Geometry check sheet. Reference: drawing and pictorial views, mm from the part's lowest x, y, z. A direction names the side the tool comes from. Coordinates: 2 decimals unless noted, no trailing zeros. Write each loop counter-clockwise with the first axis right and the second up, starting at its lowest first coordinate (ties: lowest second). Pieces come first, ordered by that corner, then holes. Notation, with made-up numbers: (75, 39.5) -> (127, 39.5) arc R8 cw to (127, 46.5) -> close; hole circle Ø1 at (64.25, -30). An arc over 180 degrees is marked (long way). Use a Markdown table: item, result.
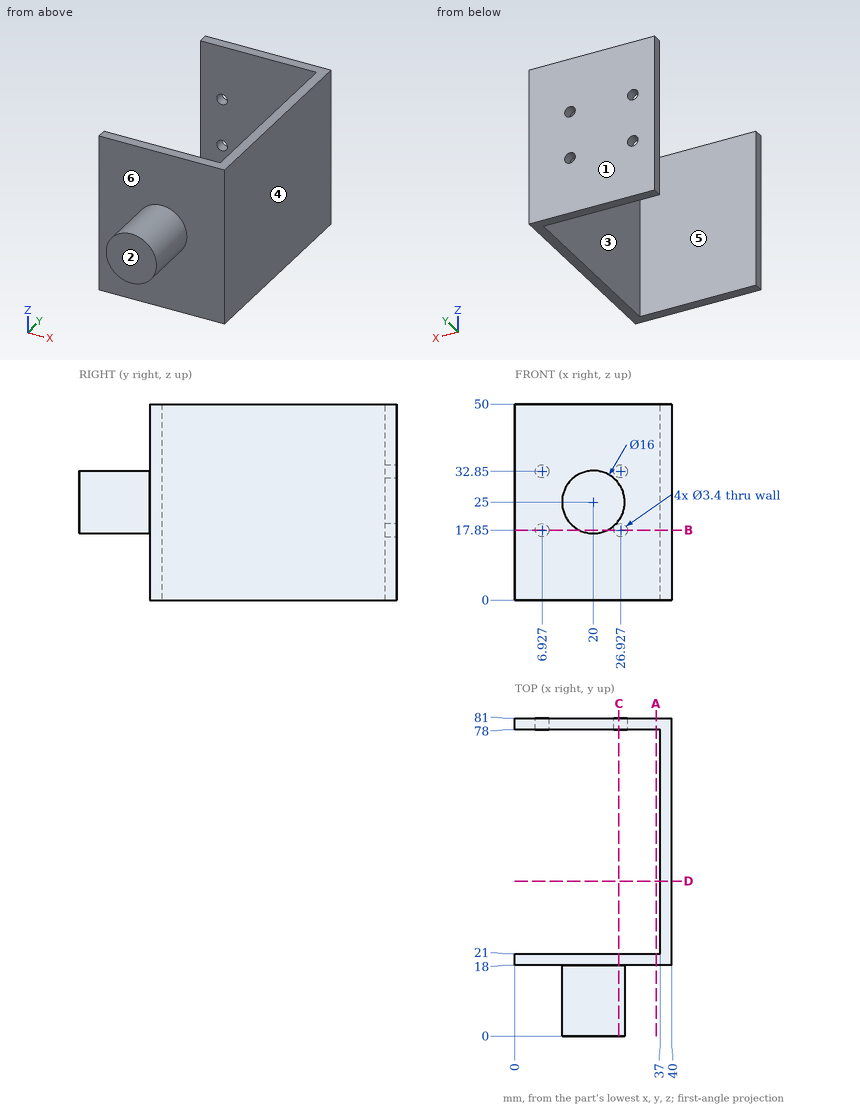
Item 1: Section check A-A on x = 36. Record the boundary of the cut face in (y, z), then the cut area to 3 significant figures.
Answer block:
| item | result |
|---|---|
| outline | (18, 0) -> (21, 0) -> (21, 50) -> (18, 50) -> close; (78, 0) -> (81, 0) -> (81, 50) -> (78, 50) -> close |
| area | 300 mm^2 |
Item 2: Section check C-C on x = 26.5. Record the boundary of the cut face in (y, z) (1 decimal).
Answer block:
| item | result |
|---|---|
| outline | (0, 20.3) -> (18, 20.3) -> (18, 0) -> (21, 0) -> (21, 50) -> (18, 50) -> (18, 29.7) -> (0, 29.7) -> close; (78, 0) -> (81, 0) -> (81, 16.2) -> (78, 16.2) -> close; (78, 19.5) -> (81, 19.5) -> (81, 31.2) -> (78, 31.2) -> close; (78, 34.5) -> (81, 34.5) -> (81, 50) -> (78, 50) -> close |
Item 3: Mould release check, pull along Y, two halves, no side actions. Record for the marked faces 1, 2, 3 and 4: +Y half, -Y half, draft (parallel to the pull), parting line (faces both ways), or undercut.
Answer block:
| item | result |
|---|---|
| face 1 | +Y half |
| face 2 | -Y half |
| face 3 | undercut |
| face 4 | draft |
Item 4: Thickness scan on L1, parallel to Y at x = 8, z = 9.5; L2, parallel to X at y = 79.7, z = 32.85; L3, parallel to X at y = 80, z = 32 (1 decimal). Record the ranges inside material, lowest first. Write a range as [from, to].
Answer block:
| item | result |
|---|---|
| L1 | y = [18, 21], [78, 81] |
| L2 | x = [0, 5.23], [8.63, 25.23], [28.63, 40] |
| L3 | x = [0, 5.5], [8.4, 25.5], [28.4, 40] |
Item 5: Depth check by flat-ended pin: P1, Ø2, axis at x = 26.93, z = 32.85, coming from the -Y side. Enter the tip coordinate at first touch or a pass-through.
Answer block:
| item | result |
|---|---|
| P1 | stops at y = 18 |
Item 6: Tool access check on the marked faces 5 and 6. Record the directions out of +Z, -Z, +X, -X, +Y, -Y that give a thin tool (end or side, any length) a straight path to the whole face; none if there is none.
Answer block:
| item | result |
|---|---|
| face 5 | +Z, -Z, -X |
| face 6 | -Y |
Item 7: Section check D-D on y = 39.5. Record the boundary of the cut face in (x, z), then the cut area to 3 significant figures.
Answer block:
| item | result |
|---|---|
| outline | (37, 0) -> (40, 0) -> (40, 50) -> (37, 50) -> close |
| area | 150 mm^2 |
Item 8: Section check B-B on z = 17.85. Record the boundary of the cut face in (x, y), then the cut area to 3 significant figures.
Answer block:
| item | result |
|---|---|
| outline | (0, 18) -> (16.41, 18) -> (16.41, 0) -> (23.59, 0) -> (23.59, 18) -> (40, 18) -> (40, 81) -> (28.63, 81) -> (28.63, 78) -> (37, 78) -> (37, 21) -> (0, 21) -> close; (0, 78) -> (5.23, 78) -> (5.23, 81) -> (0, 81) -> close; (8.63, 78) -> (25.23, 78) -> (25.23, 81) -> (8.63, 81) -> close |
| area | 520 mm^2 |
